```python
from build123d import *

# Parameters (mm, degrees)
SKETCH1_W           = 105
SKETCH1_H           = 105
BOSS_EXTRUDE1_DEPTH = 3
SKETCH3_R           = 1.15
SKETCH3_R_2         = 2.25
CUT_EXTRUDE1_DEPTH  = 75.306796459
SKETCH4_R           = 8.2
CUT_EXTRUDE2_DEPTH  = 1.6
SKETCH5_R           = 48.3
SKETCH5_R_2         = 45.3
BOSS_EXTRUDE3_DEPTH = 10
SKETCH6_R           = 12.5
CUT_EXTRUDE3_DEPTH  = 75.916620319
BOSS_EXTRUDE4_START = 40.4
SKETCH7_R           = 12.5
BOSS_EXTRUDE4_DEPTH = 40.4
FILLET1_R           = 5
SKETCH8_R           = 2.15
CUT_EXTRUDE4_DEPTH  = 10
SKETCH9_R           = 1.65
CUT_EXTRUDE5_DEPTH  = 82.412898241
FILLET2_R           = 10
SKETCH10_R          = 3.419507724
CUT_EXTRUDE6_DEPTH  = 85.526090694


with BuildPart() as part:
    # Sketch1 → Boss-Extrude1 (new body)
    with BuildSketch(Plane(origin=(0, 0, 0), x_dir=(1, 0, 0), z_dir=(0, 1, 0))):
        Rectangle(SKETCH1_W, SKETCH1_H)
    extrude(amount=BOSS_EXTRUDE1_DEPTH)

    # Sketch3 → Cut-Extrude1 (cut, through all)
    with BuildSketch(Plane(origin=(0, 3, 0), x_dir=(1, 0, 0), z_dir=(0, 1, 0))):
        with Locations(Location((-7.7, -30.2, 0), (0, 0, 270))):
            Circle(SKETCH3_R)
        with Locations(Location((7.7, -30.2, 0), (0, 0, 270))):
            Circle(SKETCH3_R)
        with Locations(Location((7.7, -14.8, 0), (0, 0, 270))):
            Circle(SKETCH3_R)
        with Locations(Location((-7.7, -14.8, 0), (0, 0, 270))):
            Circle(SKETCH3_R)
        with Locations(Location((0, -22.5, 0), (0, 0, 270))):
            Circle(SKETCH3_R_2)
    extrude(amount=-CUT_EXTRUDE1_DEPTH, mode=Mode.SUBTRACT)

    # Sketch4 → Cut-Extrude2 (cut)
    with BuildSketch(Plane(origin=(0, 3, 0), x_dir=(1, 0, 0), z_dir=(0, 1, 0))):
        with Locations(Location((0, -22.5, 0), (0, 0, 270))):
            Circle(SKETCH4_R)
    extrude(amount=-CUT_EXTRUDE2_DEPTH, mode=Mode.SUBTRACT)

    # Sketch5 → Boss-Extrude3 (add)
    with BuildSketch(Plane.XZ):
        with Locations(Location((0, 0, 0), (0, 0, 270))):
            Circle(SKETCH5_R)
        with Locations(Location((0, 0, 0), (0, 0, 270))):
            Circle(SKETCH5_R_2, mode=Mode.SUBTRACT)
    extrude(amount=BOSS_EXTRUDE3_DEPTH)

    # Sketch6 → Cut-Extrude3 (cut, through all)
    with BuildSketch(Plane.XZ):
        with Locations(Location((0, -10, 0), (0, 0, 270))):
            Circle(SKETCH6_R)
    extrude(amount=-CUT_EXTRUDE3_DEPTH, mode=Mode.SUBTRACT)

    # Sketch7 → Boss-Extrude4 (add)
    with BuildSketch(Plane.XZ.offset(BOSS_EXTRUDE4_START)):
        with BuildLine():
            ThreePointArc((-7.60254763, 3.50745237), (-16.035533906, 6.035533906), (-13.50745237, -2.39745237))
            ThreePointArc((-13.50745237, -2.39745237), (-15.5, -10), (-13.50745237, -17.60254763))
            ThreePointArc((-13.50745237, -17.60254763), (-16.035533906, -26.035533906), (-7.60254763, -23.50745237))
            ThreePointArc((-7.60254763, -23.50745237), (0, -25.5), (7.60254763, -23.50745237))
            ThreePointArc((7.60254763, -23.50745237), (16.035533906, -26.035533906), (13.50745237, -17.60254763))
            ThreePointArc((13.50745237, -17.60254763), (15.5, -10), (13.50745237, -2.39745237))
            ThreePointArc((13.50745237, -2.39745237), (16.035533906, 6.035533906), (7.60254763, 3.50745237))
            ThreePointArc((7.60254763, 3.50745237), (0, 5.5), (-7.60254763, 3.50745237))
        make_face()
        with Locations(Location((0, -10, 0), (0, 0, 270))):
            Circle(SKETCH7_R, mode=Mode.SUBTRACT)
    extrude(amount=-BOSS_EXTRUDE4_DEPTH)

    # Fillet1
    fillet1_edges = [part.edges().sort_by_distance(p)[0] for p in [
        (7.60254763, -20.2, 3.50745237),
        (-7.60254763, -20.2, 3.50745237),
        (-13.50745237, -20.2, -2.39745237),
        (-13.50745237, -20.2, -17.60254763),
        (-7.60254763, -20.2, -23.50745237),
        (7.60254763, -20.2, -23.50745237),
        (13.50745237, -20.2, -17.60254763),
        (13.50745237, -20.2, -2.39745237),
    ]]
    fillet(fillet1_edges, radius=FILLET1_R)

    # Sketch8 → Cut-Extrude4 (cut)
    with BuildSketch(Plane.XZ.offset(40.4)):
        with Locations(Location((-12.5, -22.5, 0), (0, 0, 270))):
            Circle(SKETCH8_R)
        with Locations(Location((12.5, -22.5, 0), (0, 0, 270))):
            Circle(SKETCH8_R)
        with Locations(Location((-12.5, 2.5, 0), (0, 0, 270))):
            Circle(SKETCH8_R)
        with Locations(Location((12.5, 2.5, 0), (0, 0, 270))):
            Circle(SKETCH8_R)
    extrude(amount=-CUT_EXTRUDE4_DEPTH, mode=Mode.SUBTRACT)

    # Sketch9 → Cut-Extrude5 (cut, through all)
    with BuildSketch(Plane.XZ.offset(30.4)):
        with Locations(Location((12.5, -22.5, 0), (0, 0, 270))):
            Circle(SKETCH9_R)
        with Locations(Location((-12.5, -22.5, 0), (0, 0, 270))):
            Circle(SKETCH9_R)
        with Locations(Location((-12.5, 2.5, 0), (0, 0, 270))):
            Circle(SKETCH9_R)
        with Locations(Location((12.5, 2.5, 0), (0, 0, 270))):
            Circle(SKETCH9_R)
    extrude(amount=-CUT_EXTRUDE5_DEPTH, mode=Mode.SUBTRACT)

    # Fillet2
    fillet2_edges = [part.edges().sort_by_distance(p)[0] for p in [
        (-52.5, 1.5, -52.5),
        (52.5, 1.5, -52.5),
        (52.5, 1.5, 52.5),
        (-52.5, 1.5, 52.5),
    ]]
    fillet(fillet2_edges, radius=FILLET2_R)

    # Sketch10 → Cut-Extrude6 (cut, through all)
    with BuildSketch(Plane.XZ):
        with Locations(Location((-42.5, -42.5, 0), (0, 0, 270))):
            Circle(SKETCH10_R)
        with Locations(Location((42.5, -42.5, 0), (0, 0, 270))):
            Circle(SKETCH10_R)
        with Locations(Location((42.5, 42.5, 0), (0, 0, 270))):
            Circle(SKETCH10_R)
        with Locations(Location((-42.5, 42.5, 0), (0, 0, 270))):
            Circle(SKETCH10_R)
    extrude(amount=-CUT_EXTRUDE6_DEPTH, mode=Mode.SUBTRACT)


solid = part.part
```
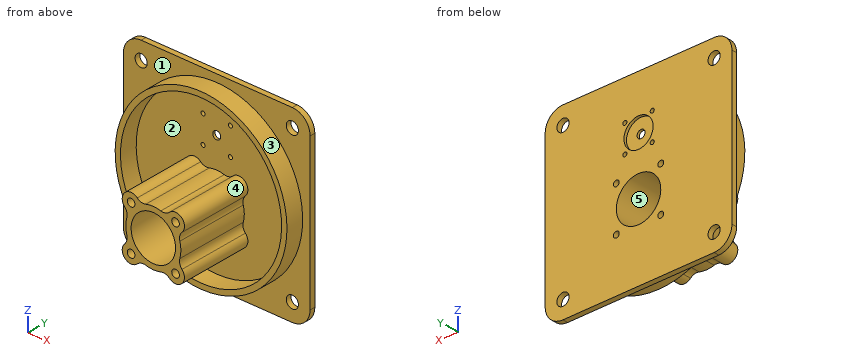
Can you work these out from the model? Positions are in its coordinate system, mm. Face numbers are marked on the shaded views. A direction names the side the tool comes from. Coordinates: 2 decimals unless noted, no trailing zeros. Write each loop counter-clockwise with the first axis right and the second up, starting at its lowest first coordinate (ties: lowest second). Pieces come first, ordered by that corner, then holes. Notation, with made-up numbers: M 5.5,-20 L 55.5,-20 A18 cw 55.5,-6 Z; hole C 12,50.25 d4. An arc over 180 degrees is marked long. Write item = value, one per line. Start each with the question number.
Q1. If we section it at D-D, the plane y = -33: State how many separate pieces and enclosed holes the cut face has, then the cut area to 3 significant figures.
Q2. On a 3-axis mill with a long thin cutter (end or side, diameter ignored), from which of +Z, -Z, +X, -X, +Y, -Y can I reach the whole of each face in a straight line? I mean the marked faces 4 and 5. Say none if no direction works.
Q3. If we section it at B-B, the plane z = -8.5: Write out the boundary of the cut face in (x, y), then the cut area to 3 significant figures.
Q4. If we section it at C-C, the plane x = -33: Write out the boundary of the cut face in (y, z).
Q5. If I drill on L1, parallel to Z at x = 42, y = 1; L2, parallel to X at y = -8, z = -10; L3, parallel to X at y = 0.6, z = -42.5, over which ranges is the centre line in solid material (lowest first)? Write a range as [from, to].
Q6. If we section it at A-A, the plane x = 44: Write out the boundary of the cut face in (y, z), then the cut area to 3 significant figures.
Q7. Thinking about a two-plate mould opening in X: for the marked faces 1, 2 and 3, which applies, released by +X, released by -X, zero draft, split by the parting line, or undercut?
Q8. I'm going to push flat-ended pins straight in: pin 1 (5 mm diameter, centred on y = -31.5, z = -23.5, fed in from -X); pin 2 (1.5 mm diameter, centred on x = -33.5, z = 16, fed in from -Y); pin 3 (1.5 mm diameter, centred on y = -2.5, z = -37.5, fed in from -X). Where does each tip first touch, or does it pass through?
Check sheet entries:
q1.separate_pieces = 1
q1.enclosed_holes = 5
q1.area = 474 mm²
q2.face_4 = -Y
q2.face_5 = +Y, -Y
q3.outline = M -52.5,0 L -47.55,0 L -47.55,-10 L -44.5,-10 L -44.5,0 L -15.43,0 L -15.43,-40.4 L -12.41,-40.4 L -12.41,3 L -52.5,3 Z; M 12.41,-40.4 L 15.43,-40.4 L 15.43,0 L 44.5,0 L 44.5,-10 L 47.55,-10 L 47.55,0 L 52.5,0 L 52.5,3 L 12.41,3 Z
q3.area = 545 mm²
q4.outline = M -10,-35.27 L 0,-35.27 L 0,-52.5 L 3,-52.5 L 3,52.5 L 0,52.5 L 0,35.27 L -10,35.27 L -10,31.03 L 0,31.03 L 0,-31.03 L -10,-31.03 Z
q5.L1 = [-52.5, -45.88], [-39.12, 39.12], [45.88, 52.5]
q5.L2 = [-47.25, -44.18], [-15.5, -12.5], [12.5, 15.5], [44.18, 47.25]
q5.L3 = [-52.5, -45.92], [-39.08, 39.08], [45.92, 52.5]
q6.outline = M -10,-19.92 L 0,-19.92 L 0,-39.43 L 3,-39.43 L 3,39.43 L 0,39.43 L 0,19.92 L -10,19.92 L -10,10.77 L 0,10.77 L 0,-10.77 L -10,-10.77 Z; M 0,-52.39 L 3,-52.39 L 3,-45.57 L 0,-45.57 Z; M 0,45.57 L 3,45.57 L 3,52.39 L 0,52.39 Z
q6.area = 460 mm²
q7.face_1 = zero draft
q7.face_2 = undercut
q7.face_3 = split by the parting line
q8.pin_1 = -17.5
q8.pin_2 = 0
q8.pin_3 = -31.34
